Geometry check sheet. Reference: the model listing, model coordinates, mm. Face numbers are marked on the shaded views. A direction names the side the tool comes from. Round coordinates to 2 decimals unless told otherwise and drop trailing zeros. Write each loop counter-clockwise with the first axis right and the second up, starting at its lowest first coordinate (ties: lowest second). Pieces come first, ordered by that corner, then holes. Notation, with made-up numbers: M 19.25,84 L 44.25,84 A12 ccw 44.25,102 Z; hole C -27.5,11 d9. An arc over 180 degrees is marked long. Use a Markdown table: item, result.
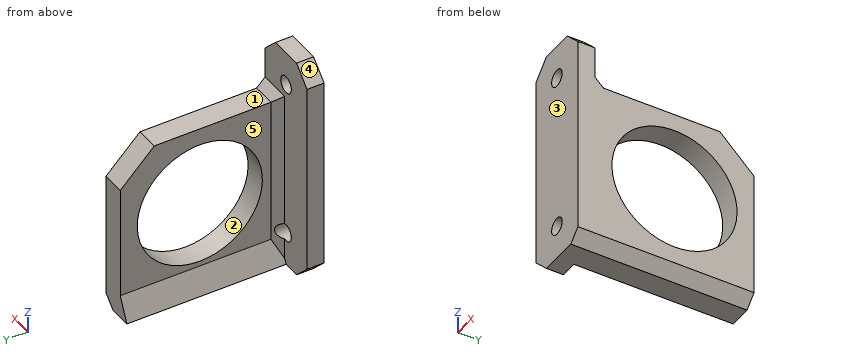
```python
from build123d import *

# Parameters (mm, degrees)
SKETCH1_R           = 1.5
BOSS_EXTRUDE1_DEPTH = 3
BOSS_EXTRUDE2_DEPTH = 28
CHAMFER1_SIZE       = 2
SKETCH4_R           = 11
CUT_EXTRUDE1_DEPTH  = 11
CHAMFER2_SIZE       = 6
CHAMFER3_SIZE       = 1.5


with BuildPart() as part:
    # Sketch1 → Boss-Extrude1 (new body)
    with BuildSketch(Plane(origin=(0, 0, 0), x_dir=(1, 0, 0), z_dir=(0, 1, 0))):
        Polygon((-6, 17), (-3, 20), (6, 20), (6, -17), (3, -20), (-3, -20), (-6, -17), align=None)
        with Locations(Location((0, 14, 0), (0, 0, 270))):
            Circle(SKETCH1_R, mode=Mode.SUBTRACT)
        with Locations(Location((0, -14, 0), (0, 0, 270))):
            Circle(SKETCH1_R, mode=Mode.SUBTRACT)
    extrude(amount=BOSS_EXTRUDE1_DEPTH)

    # Sketch2 → Boss-Extrude2 (add)
    with BuildSketch(Plane(origin=(0, 3, 0), x_dir=(1, 0, 0), z_dir=(0, 1, 0))):
        Polygon((6, -10), (6, 20), (0, 20), (1.9, 15.9), (1.9, -10), align=None)
    extrude(amount=BOSS_EXTRUDE2_DEPTH)

    # Chamfer1
    chamfer1_edges = [part.edges().sort_by_distance(p)[0] for p in [
        (6, 15.5, -20),
    ]]
    chamfer(chamfer1_edges, length=CHAMFER1_SIZE)

    # Sketch4 → Cut-Extrude1 (cut)
    with BuildSketch(Plane(origin=(6, 0, 0), x_dir=(0, 0, -1), z_dir=(1, 0, 0))):
        with Locations((4, 17)):
            Circle(SKETCH4_R)
    extrude(amount=-CUT_EXTRUDE1_DEPTH, mode=Mode.SUBTRACT)

    # Chamfer2
    chamfer2_edges = [part.edges().sort_by_distance(p)[0] for p in [
        (3.95, 31, 10),
    ]]
    chamfer(chamfer2_edges, length=CHAMFER2_SIZE)

    # Chamfer3
    # the kernel refuses this chamfer: 1.5 mm, written as the material it adds along each edge
    with BuildSketch(Plane(origin=(1.9, 3, 10), x_dir=(0, 0.9996219169112968, -0.02749587661058678), z_dir=(1, 0, 0))) as chamfer3_piece_1:
        Polygon((CHAMFER3_SIZE * 0.999621916911, CHAMFER3_SIZE * 0.0274958766106), (-CHAMFER3_SIZE * 0.0274958766106, CHAMFER3_SIZE * 0.999621916911), (0, 0), align=None)
    extrude(amount=4.1)
    with BuildSketch(Plane(origin=(1.9, 3, -19.757524482), x_dir=(0.02749587661058635, 0.9996219169112968, 0), z_dir=(0, 0, 1))) as chamfer3_piece_2_section:
        Polygon((CHAMFER3_SIZE * 0.999621916911, CHAMFER3_SIZE * 0.0274958766106), (-CHAMFER3_SIZE * 0.0274958766106, CHAMFER3_SIZE * 0.999621916911), (0, 0), align=None)
    chamfer3_piece_2 = extrude(amount=29.757524482, mode=Mode.PRIVATE)
    chamfer3_piece_2 = chamfer3_piece_2 - Plane(origin=(0, 3.553768572, -14), x_dir=(0, 0, 1), z_dir=(0, -1, 0)) * Cylinder(1.5, 66, mode=Mode.PRIVATE)
    add(chamfer3_piece_2)
    with BuildSketch(Plane(origin=(1.9, 3, -19.757524482), x_dir=(0.02749587661058635, 0.9996219169112968, 0), z_dir=(0, 0, 1))) as chamfer3_piece_3a_section:
        Polygon((CHAMFER3_SIZE * 0.999621916911, CHAMFER3_SIZE * 0.0274958766106), (-CHAMFER3_SIZE * 0.0274958766106, CHAMFER3_SIZE * 0.999621916911), (0, 0), align=None)
    chamfer3_piece_3a = extrude(amount=33.615048964, mode=Mode.PRIVATE)
    chamfer3_piece_3a = split(chamfer3_piece_3a, bisect_by=Plane(origin=(1.452851003, 3.519674643, 10), z_dir=(0, 0, 1)), keep=Keep.TOP, mode=Mode.PRIVATE)
    chamfer3_piece_3a = chamfer3_piece_3a - Plane(origin=(0, 3.519674643, 14), x_dir=(0, 0, 1), z_dir=(0, -1, 0)) * Cylinder(1.5, 74, mode=Mode.PRIVATE)
    with BuildSketch(Plane(origin=(-1.957524482, 3, 10), x_dir=(0, 0.9996219169112968, -0.02749587661058678), z_dir=(1, 0, 0))) as chamfer3_piece_3b_section:
        Polygon((CHAMFER3_SIZE * 0.999621916911, CHAMFER3_SIZE * 0.0274958766106), (-CHAMFER3_SIZE * 0.0274958766106, CHAMFER3_SIZE * 0.999621916911), (0, 0), align=None)
    chamfer3_piece_3b = extrude(amount=7.957524482, mode=Mode.PRIVATE)
    chamfer3_piece_3b = split(chamfer3_piece_3b, bisect_by=Plane(origin=(1.9, 3.49469044, 10.49469044), z_dir=(-1, 0, 0)), keep=Keep.TOP, mode=Mode.PRIVATE)
    chamfer3_piece_3 = chamfer3_piece_3a & chamfer3_piece_3b
    add(chamfer3_piece_3)


solid = part.part
```
Item 1: Cross-section at A-A, the plane y = 17. Record the cut outline in (x, z), and give its area (3 significant figures).
Outcome:
| item | result |
|---|---|
| outline | M 0,-20 L 4,-20 L 6,-18 L 6,-15 L 1.9,-15 L 1.9,-15.9 Z; M 1.9,7 L 6,7 L 6,10 L 1.9,10 Z |
| area | 34.7 mm2 |
Item 2: Cross-section at C-C, the plane x = 4.5. Record the cut outline in (y, z).
Outcome:
| item | result |
|---|---|
| outline | M 0,-19.5 L 31,-19.5 L 31,4 L 25,10 L 4.5,10 L 3,11.5 L 3,18.5 L 0,18.5 Z; hole C 17,-4 d22 |
Item 3: Material ranges on line 1 along Y through (x, z) = (3.95, -4); line 2 along Y through (x, z) = (-0.25, -6.5); line 3 along X through (y, z) = (21, 8.5), recorded low to high. Write a range as from..to.
Outcome:
| item | result |
|---|---|
| line 1 | y = 0..6, 28..31 |
| line 2 | y = 0..3 |
| line 3 | x = 1.9..6 |
Item 4: Access from +Z, -Z, +X, -X, +Y, -Y to the whole of each face (thin tool, end or side, straight path). Record for the marked faces 4 and 5.
Outcome:
| item | result |
|---|---|
| face 4 | +Z, -X, +Y, -Y |
| face 5 | +Z, -X, +Y |
Item 5: Cross-section at B-B, the plane z = -4. Record the cut outline in (x, y), and give its area (3 significant figures).
Outcome:
| item | result |
|---|---|
| outline | M -6,0 L 6,0 L 6,6 L 1.9,6 L 1.9,4.5 L 0.4,3 L -6,3 Z; M 1.9,28 L 6,28 L 6,31 L 1.9,31 Z |
| area | 61.7 mm2 |
Item 6: Go/stop test with flat-tipped pins: pin 1 (6 mm diameter, centred on x = 2, z = 8, fed in from +Y); pin 2 (1 mm diameter, centred on x = -4, z = -11.5, fed in from +Y); pin 3 (1.5 mm diameter, centred on y = 16.5, z = -15, fed in from -X). Record where each tip stops, or that it passes through.
Outcome:
| item | result |
|---|---|
| pin 1 | stops at y = 30 |
| pin 2 | stops at y = 3 |
| pin 3 | stops at x = 1.9 |
Item 7: Cross-section at D-D, the plane z = -13. Record the cut outline in (x, y), and give its area (3 significant figures).
Outcome:
| item | result |
|---|---|
| outline | M -6,0 L -1.12,0 L -1.12,3 L -6,3 Z; M 1.12,0 L 6,0 L 6,10.68 L 1.9,10.68 L 1.9,4.5 L 1.12,3.72 Z; M 1.9,23.32 L 6,23.32 L 6,31 L 1.9,31 Z |
| area | 93.1 mm2 |
Item 8: Mould release check, pull along Z, two halves, no side actions. Record for the marked faces 1, 2 and 3: +Z half, -Z half, draft (parallel to the pull), parting line (faces both ways), or undercut.
Outcome:
| item | result |
|---|---|
| face 1 | +Z half |
| face 2 | undercut |
| face 3 | draft |
